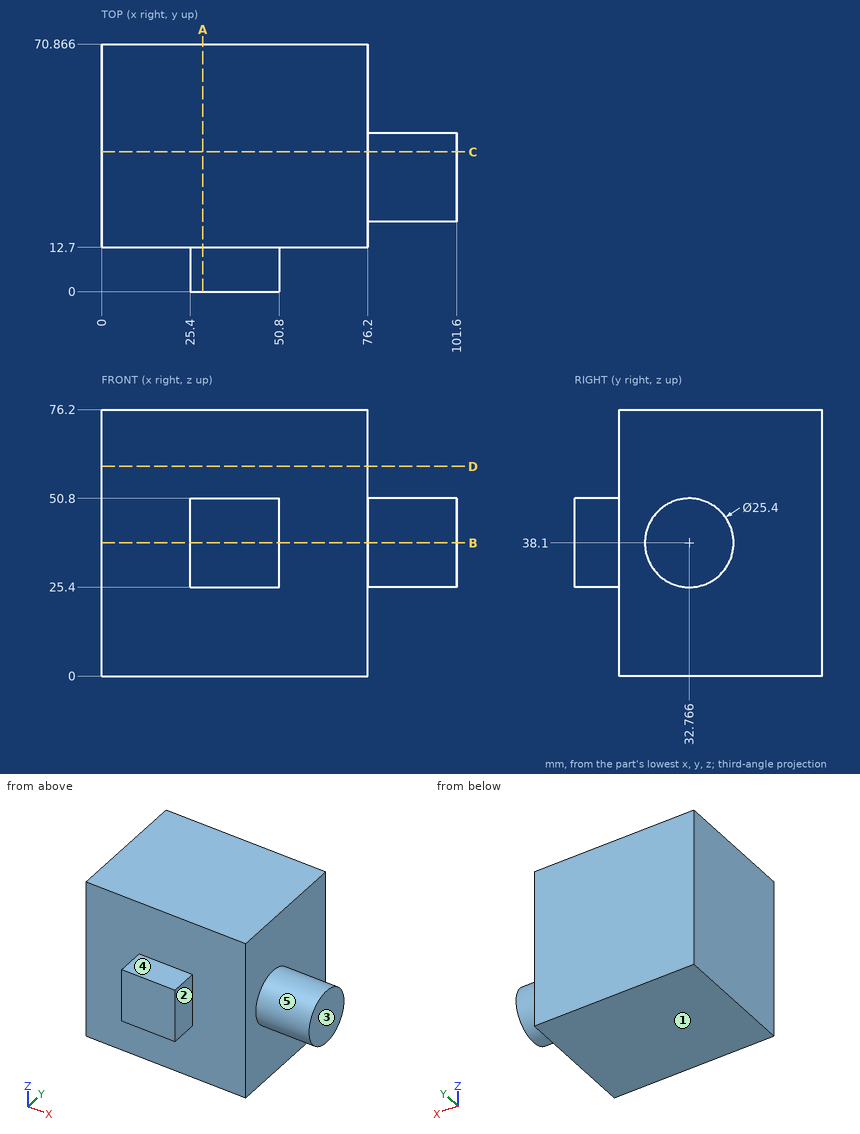
Can you work these out from the drawing? Everything is in mm from the part's minimum corner. A direction names the side the tool comes from. Coordinates: 2 decimals unless noted, no trailing zeros. Write each loop counter-clockwise with the first axis right and the second up, starting at its lowest first coordinate (ties: lowest second). Pieces come first, ordered by that corner, then holes. Notation, with made-up numbers: (-19.75, -11.5) - (13.25, -11.5) arc R11 cw to (13.25, -6.5) - close; hole circle Ø8 at (-23.5, 84). An arc over 180 degrees is marked (long way). One line per item, written item: value.
1) Suppose I cut it at D-D on z = 60. Write out the boundary of the cut face in (x, y), and give its area (3 significant figures).
Model answer:
outline: (0, 12.7) - (76.2, 12.7) - (76.2, 70.87) - (0, 70.87) - close
area: 4,430 mm²
2) On a 3-axis mill with a long thin cutter (end or side, diameter ignored), from which of +Z, -Z, +X, -X, +Y, -Y can I reach the whole of each face in a straight line? I mean the marked faces 1, 2, 3, 4 and 5. Say none if no direction works.
Model answer:
face 1: -Z, +X, -X, +Y, -Y
face 2: +Z, -Z, +X, -Y
face 3: +Z, -Z, +X, +Y, -Y
face 4: +Z, +X, -X, -Y
face 5: +X
3) I'm going to push flat-ended pins straight in: P1, Ø4, axis at x = 71.5, y = 37.5, coming from the -Z side; P2, Ø14, axis at x = 40.5, y = 4, coming from the -Z side; P3, Ø3, axis at y = 41, z = 61, coming from the +X side; P4, Ø4, axis at y = 8, z = 43.5, coming from the -X side. Where does each tip first touch, or does it pass through?
Model answer:
P1: stops at z = 0
P2: stops at z = 25.4
P3: stops at x = 76.2
P4: stops at x = 25.4
4) Suppose I cut it at A-A on x = 29. Write out the boundary of the cut face in (y, z), and give its area (3 significant figures).
Model answer:
outline: (0, 25.4) - (12.7, 25.4) - (12.7, 0) - (70.87, 0) - (70.87, 76.2) - (12.7, 76.2) - (12.7, 50.8) - (0, 50.8) - close
area: 4,750 mm²
5) Suppose I cut it at B-B on z = 38.1. Write out the boundary of the cut face in (x, y).
Model answer:
outline: (0, 12.7) - (25.4, 12.7) - (25.4, 0) - (50.8, 0) - (50.8, 12.7) - (76.2, 12.7) - (76.2, 20.07) - (101.6, 20.07) - (101.6, 45.47) - (76.2, 45.47) - (76.2, 70.87) - (0, 70.87) - close
6) Suppose I cut it at C-C on y = 40. Write out the boundary of the cut face in (x, z).
Model answer:
outline: (0, 0) - (76.2, 0) - (76.2, 27.66) - (101.6, 27.66) - (101.6, 48.54) - (76.2, 48.54) - (76.2, 76.2) - (0, 76.2) - close
7) I need wall thicknesses on line 1 along Z through (x, y) = (26.5, 9.5); line 2 along Y through (x, z) = (51, 26.5); line 3 along X through (y, z) = (20, 8.5). Which ranges of each line are inside material? Lowest first, please.
Model answer:
line 1: z = 25.4 to 50.8
line 2: y = 12.7 to 70.87
line 3: x = 0 to 76.2
